Part model, mm, in its own coordinate system. Face numbers are marked on the shaded views. Give positions to 0.01 mm unless a question says otherwise; leave off trailing zeros. Write each loop counter-clockwise with the first axis right and the second up, starting at its lowest first coordinate (ties: lowest second). Pieces come first, ordered by that corner, then holes. Notation, with made-up numbers: (51, -28.5) - (66, -28.5) arc R29 ccw to (66, 9.5) - close; hole circle Ø6 at (69.25, 51). An arc over 180 degrees is marked (long way). Answer as a JSON object with one key per item and string values. Group by question number.
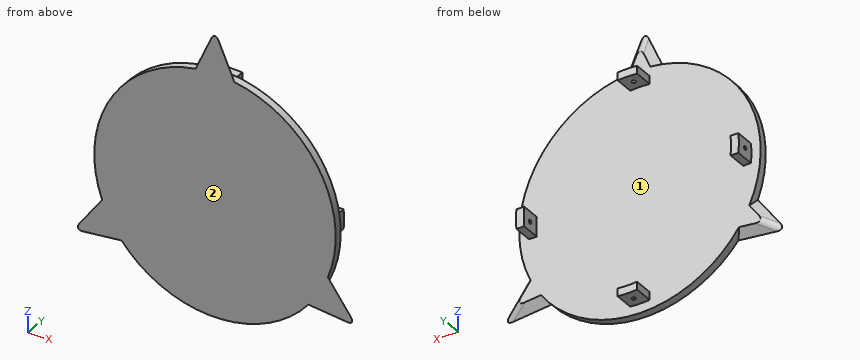
```python
from build123d import *

# Parameters (mm, degrees)
SKETCH4_R            = 61.9125
BOSS_EXTRUDE1_DEPTH  = 4
BOSS_EXTRUDE2_DEPTH  = 10
M2_CLEARANCE_HOLE2_D = 2
M2_CLEARANCE_HOLE3_D = 2
BOSS_EXTRUDE3_DEPTH  = 4
CHAMFER1_SIZE        = 4
FILLET1_R            = 3


# Some blends are built 0.0001 mm under size
with BuildPart() as part:
    # Sketch4 → Boss-Extrude1 (new body)
    with BuildSketch(Plane(origin=(0, 0, 0), x_dir=(1, 0, 0), z_dir=(0, 1, 0))):
        with Locations(Location((0, 0, 0), (0, 0, 270))):
            Circle(SKETCH4_R)
    extrude(amount=-BOSS_EXTRUDE1_DEPTH)

    # Sketch15 → Boss-Extrude2 (add)
    with BuildSketch(Plane(origin=(0, 0, 0), x_dir=(1, 0, 0), z_dir=(0, 1, 0))):
        with BuildLine():
            Line((-52.91429391, -5), (-56.930857187, -5))
            ThreePointArc((-56.930857187, -5), (-57.15, 0), (-56.930857187, 5))
            Line((-56.930857187, 5), (-52.91429391, 5))
            ThreePointArc((-52.91429391, 5), (-53.15, 0), (-52.91429391, -5))
        make_face()
        with BuildLine():
            Line((-5, 52.91429391), (-5, 56.930857187))
            ThreePointArc((-5, 56.930857187), (0, 57.15), (5, 56.930857187))
            Line((5, 56.930857187), (5, 52.91429391))
            ThreePointArc((5, 52.91429391), (0, 53.15), (-5, 52.91429391))
        make_face()
        with BuildLine():
            Line((-5, -52.91429391), (-5, -56.930857187))
            ThreePointArc((-5, -56.930857187), (0, -57.15), (5, -56.930857187))
            Line((5, -56.930857187), (5, -52.91429391))
            ThreePointArc((5, -52.91429391), (0, -53.15), (-5, -52.91429391))
        make_face()
        with BuildLine():
            Line((52.91429391, 5), (56.930857187, 5))
            ThreePointArc((56.930857187, 5), (57.15, 0), (56.930857187, -5))
            Line((56.930857187, -5), (52.91429391, -5))
            ThreePointArc((52.91429391, -5), (53.15, 0), (52.91429391, 5))
        make_face()
    extrude(amount=BOSS_EXTRUDE2_DEPTH)

    # M2 Clearance Hole2 (through all)
    with Locations(Plane(origin=(0, 5, 57.15), x_dir=(1, 0, 0), z_dir=(0, 0, 1))):
        with Locations((0, 0)):
            Hole(M2_CLEARANCE_HOLE2_D / 2)

    # M2 Clearance Hole3 (through all)
    with Locations(Plane(origin=(57.15, 5, 0), x_dir=(0, 0, 1), z_dir=(1, 0, 0))):
        with Locations((0, 0)):
            Hole(M2_CLEARANCE_HOLE3_D / 2)

    # Sketch19 → Boss-Extrude3 (add)
    with BuildSketch(Plane(origin=(0, 0, 0), x_dir=(1, 0, 0), z_dir=(0, 1, 0))):
        with BuildLine():
            Line((9.967336465, -61.104908641), (0, -83.564835105))
            Line((0, -83.564835105), (-9.967336465, -61.104908641))
            ThreePointArc((-9.967336465, -61.104908641), (0, -61.9125), (9.967336465, -61.104908641))
        make_face()
        with BuildLine():
            Line((-47.934734947, 39.184420907), (-72.369270064, 41.782417553))
            Line((-72.369270064, 41.782417553), (-57.902071411, 21.920487734))
            ThreePointArc((-57.902071411, 21.920487734), (-53.617797812, 30.95625), (-47.934734947, 39.184420907))
        make_face()
        with BuildLine():
            Line((57.902071411, 21.920487734), (72.369270064, 41.782417553))
            Line((72.369270064, 41.782417553), (47.934734947, 39.184420907))
            ThreePointArc((47.934734947, 39.184420907), (53.617797812, 30.95625), (57.902071411, 21.920487734))
        make_face()
    extrude(amount=-BOSS_EXTRUDE3_DEPTH)

    # Chamfer1
    chamfer1_edges = [part.edges().sort_by_distance(p)[0] for p in [
        (-60.152002506, 0, -40.48341923),
        (-65.135670738, 0, -31.851452643),
        (60.152002506, 0, -40.48341923),
        (65.135670738, 0, -31.851452643),
        (4.983668232, 0, 72.334871873),
        (-4.983668232, 0, 72.334871873),
    ]]
    chamfer(chamfer1_edges, length=CHAMFER1_SIZE - 0.0001)  # a hair under: the kernel refuses the full size

    # Fillet1
    # the kernel refuses this fillet: 3 mm, written as the material it takes off along each edge
    with BuildSketch(Plane(origin=(-58.731491813, 2.387836055, -33.908642608), x_dir=(-0.1711376698055133, -0.5989233275147531, 0.7823060435227348), z_dir=(-0.8025159588326043, -0.3758867485808155, -0.46333280486096456)), Plane(origin=(58.731491813, 2.387836055, -33.908642608), x_dir=(-0.5919280723220329, -0.5989233275147517, -0.5393625913574092), z_dir=(0.80251595883259, -0.3758867485808147, -0.4633328048609902))) as fillet1_piece_1:
        with BuildLine():
            CenterArc((FILLET1_R * 0.847005492593, -FILLET1_R), FILLET1_R, 90, 80.529565024)
            Line((-FILLET1_R * 0.139365143358, -FILLET1_R * 0.835461346383), (0, 0))
            Line((0, 0), (FILLET1_R * 0.847005492593, 0))
        make_face()
    extrude(amount=23.346319451, mode=Mode.SUBTRACT)
    with BuildSketch(Plane(origin=(0, 2.387836055, 67.817285216), x_dir=(-0.7630657421275423, -0.5989233275147525, -0.24294345216531282), z_dir=(0, -0.37588674858081544, 0.9266656097219444))) as fillet1_piece_2:
        with BuildLine():
            CenterArc((FILLET1_R * 0.847005492593, FILLET1_R), FILLET1_R, 189.470434976, 80.529565024)
            Line((-FILLET1_R * 0.139365143358, FILLET1_R * 0.835461346383), (0, 0))
            Line((0, 0), (FILLET1_R * 0.847005492593, 0))
        make_face()
    extrude(amount=23.346319451, mode=Mode.SUBTRACT)


solid = part.part
```
1) Drop flat-ended pins along their axis: P1, Ø2, axis at y = 5.5, z = -54.5, coming from the +X side; P2, Ø3, axis at y = 5, z = -55, coming from the -X side; P3, Ø8, axis at x = -15.5, y = 2.5, coming from the +Z side; P4, Ø1.5, axis at x = -24.5, y = 1, coming from the +Z side. Give the stop position or say it passes through.
2) Band-saw the part on A-A (y = 2.25). List the corners of the cut face in (x, z).
3) Probe line 1 (Z direction, x = 56.3, y = 5); line 2 (Y direction, x = -54.1, z = 0). List the from-to ranges inside material, lowest first.
4) Mould opens along Y. For the marked faces 1 and 2 say: pulls with the +Y half, pulls with the -Y half, needs draft (parallel to the pull), parting line crosses it, or undercut.
5) Band-saw the part on B-B (x = 46). List the corners of the cut face in (y, z).
6) Band-saw the part on C-C (x = -29). List the corners of the cut face in (y, z).
Verdict:
{
 "1": {"P1": "x = 5", "P2": "x = -5", "P3": "z = 60.66", "P4": "through"},
 "2": {"outline": "(-56.93, -5) - (-52.91, -5) arc R53.15 cw to (-52.91, 5) - (-56.93, 5) arc R57.15 ccw to start; (-5, -56.93) arc R57.15 ccw to (5, -56.93) - (5, -52.91) arc R53.15 cw to (-5, -52.91) - close; (-5, 52.91) arc R53.15 cw to (5, 52.91) - (5, 56.93) arc R57.15 ccw to (-5, 56.93) - close; (52.91, -5) - (56.93, -5) arc R57.15 ccw to (56.93, 5) - (52.91, 5) arc R53.15 cw to start"},
 "3": {"line 1": "-5 to -1, 1 to 5", "line 2": "-4 to 4, 6 to 10"},
 "4": {"face 1": "pulls with the +Y half", "face 2": "pulls with the -Y half"},
 "5": {"outline": "(-4, -41.44) - (0, -41.44) - (0, 41.44) - (-4, 41.44) - close"},
 "6": {"outline": "(-4, -54.7) - (0, -54.7) - (0, 54.7) - (-4, 54.7) - close"}
}
